The figure shows three views and two pictorial views of one solid part (mm, origin at its lowest corner). Answer the questions. A direction names the side the tool comes from. Give positions to 0.01 mm unless a question says otherwise; leave off trailing zeros. Order: outer loops, then holes, each group sorted by start corner. A loop starts at its lowest first (then second) coordinate and runs counter-clockwise, first axis right, second up. Notation, with made-up numbers: M -30,27.5 L -6,27.5 A11 ccw -6,45.5 Z; hole C 61.25,1.5 d7. An arc over 180 degrees is marked long. One line per item, written item: value.
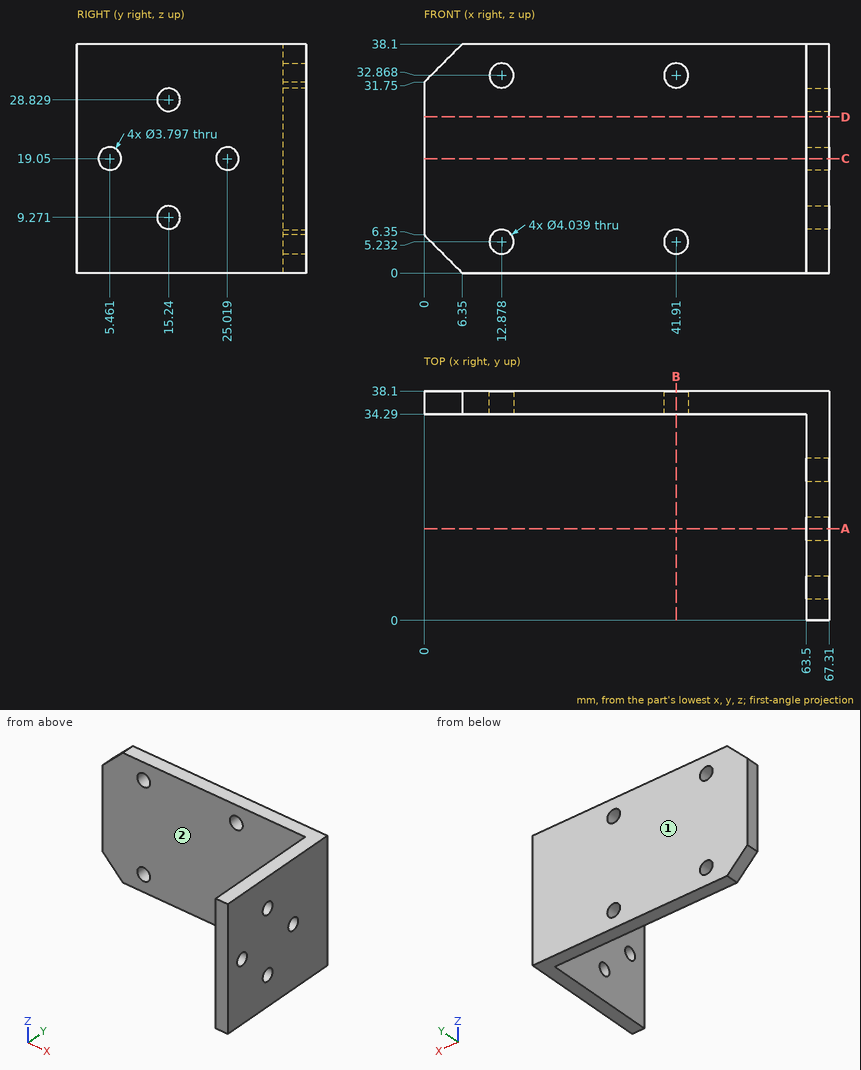
1) Which of the six approach directions +Z, -Z, +X, -X, +Y, -Y give full straight-line access (tool end or side, diameter ignored) to the marked faces 1 and 2?
Reported:
face 1: +Z, -Z, +X, -X, +Y
face 2: +Z, -Z, -X, -Y
2) Find section D-D, the plane z = 26. Write down the section's boundary in (x, y), plus the area to 3 significant figures.
Reported:
outline: M 0,34.29 L 63.5,34.29 L 63.5,0 L 67.31,0 L 67.31,38.1 L 0,38.1 Z
area: 387 mm^2
3) Find section C-C, the plane z = 19.05. Write down the section's boundary in (x, y).
Reported:
outline: M 0,34.29 L 63.5,34.29 L 63.5,26.92 L 67.31,26.92 L 67.31,38.1 L 0,38.1 Z; M 63.5,0 L 67.31,0 L 67.31,3.56 L 63.5,3.56 Z; M 63.5,7.36 L 67.31,7.36 L 67.31,23.12 L 63.5,23.12 Z
4) Find section B-B, the plane x = 41.91. Write down the section's boundary in (y, z), plus the area to 3 significant figures.
Reported:
outline: M 34.29,0 L 38.1,0 L 38.1,3.21 L 34.29,3.21 Z; M 34.29,7.25 L 38.1,7.25 L 38.1,30.85 L 34.29,30.85 Z; M 34.29,34.89 L 38.1,34.89 L 38.1,38.1 L 34.29,38.1 Z
area: 114 mm^2
5) Find section A-A, the plane y = 15.24. Write down the section's boundary in (x, z), plus the area to 3 significant figures.
Reported:
outline: M 63.5,0 L 67.31,0 L 67.31,7.37 L 63.5,7.37 Z; M 63.5,11.17 L 67.31,11.17 L 67.31,26.93 L 63.5,26.93 Z; M 63.5,30.73 L 67.31,30.73 L 67.31,38.1 L 63.5,38.1 Z
area: 116 mm^2
6) Each of these flat-tipped pins is pushed along its axis until it touches: pin 1 Ø4.5 at (y, z) = (15.24, 28.829) entering from +X; pin 2 Ø5.5 at (x, z) = (41.91, 32.87) entering from -Y; pin 3 Ø8 at (y, z) = (8, 20.5) entering from -X. Where does it stop, or does it pass through?
Reported:
pin 1: stops at x = 67.31
pin 2: stops at y = 34.29
pin 3: stops at x = 63.5
7) Consider probe 1 along Z at (x, y) = (41.91, 37); probe 2 along Z at (x, y) = (64.65, 15.24); probe 3 along Y at (x, z) = (66, 19). Determine where each line is inside the solid, lowest interval first.
Reported:
probe 1: z = 0 to 3.21, 7.25 to 30.85, 34.89 to 38.1
probe 2: z = 0 to 7.37, 11.17 to 26.93, 30.73 to 38.1
probe 3: y = 0 to 3.56, 7.36 to 23.12, 26.92 to 38.1
